```python
from build123d import *

# Parameters (mm, degrees)
SKETCH1_W                = 15.875
SKETCH1_H                = 15.875
BOSS_EXTRUDE1_DEPTH      = 25.4
BOSS_EXTRUDE3_DEPTH      = 3.175
BOSS_EXTRUDE3_DEPTH_BACK = 3.175
SKETCH4_R                = 1.190625
CUT_EXTRUDE1_DEPTH       = 16.875
SKETCH8_R                = 1.5875
CUT_EXTRUDE3_DEPTH       = 7.9375
SKETCH7_R                = 1.5875
CUT_EXTRUDE4_DEPTH       = 7.9375
SKETCH9_W                = 9.525
SKETCH9_H                = 4.7625
CUT_EXTRUDE5_DEPTH       = 26.4
CUT_EXTRUDE6_DEPTH       = 12.1125


with BuildPart() as part:
    # Sketch1 → Boss-Extrude1 (new body)
    with BuildSketch(Plane.XY):
        Rectangle(SKETCH1_W, SKETCH1_H)
    extrude(amount=BOSS_EXTRUDE1_DEPTH)

    # Sketch3 → Boss-Extrude3 (add, two sides)
    with BuildSketch(Plane(origin=(0, 0, 0), x_dir=(1, 0, 0), z_dir=(0, 1, 0))) as boss_extrude3_sk:
        with BuildLine():
            Line((-7.9375, 0), (7.9375, 0))
            ThreePointArc((7.9375, 0), (0, 7.9375), (-7.9375, 0))
        make_face()
    extrude(amount=BOSS_EXTRUDE3_DEPTH)
    extrude(boss_extrude3_sk.sketch, amount=-BOSS_EXTRUDE3_DEPTH_BACK)

    # Sketch4 → Cut-Extrude1 (cut, through all)
    with BuildSketch(Plane(origin=(7.9375, 0, 0), x_dir=(0, 0, -1), z_dir=(1, 0, 0))):
        with Locations((-12.7, 0)):
            Circle(SKETCH4_R)
    extrude(amount=-CUT_EXTRUDE1_DEPTH, mode=Mode.SUBTRACT)

    # Sketch8 → Cut-Extrude3 (cut)
    with BuildSketch(Plane(origin=(6.380613831, 0, -4.72140587), x_dir=(-0.594822787, 0, -0.803856861), z_dir=(0.803856861, 0, -0.594822787))):
        Circle(SKETCH8_R)
    extrude(amount=-CUT_EXTRUDE3_DEPTH, mode=Mode.SUBTRACT)

    # Sketch7 → Cut-Extrude4 (cut)
    with BuildSketch(Plane(origin=(-4.72140587, 0, -6.380613831), x_dir=(0.803856861, 0, -0.594822787), z_dir=(0.594822787, 0, 0.803856861))):
        Circle(SKETCH7_R)
    extrude(amount=CUT_EXTRUDE4_DEPTH, mode=Mode.SUBTRACT)

    # Sketch9 → Cut-Extrude5 (cut, through all)
    with BuildSketch(Plane(origin=(0, 0, 0), x_dir=(-1, 0, 0), z_dir=(0, 0, -1))):
        with Locations((0, 5.55625)):
            Rectangle(SKETCH9_W, SKETCH9_H)
        with Locations((0, -5.55625)):
            Rectangle(SKETCH9_W, SKETCH9_H)
    extrude(amount=-CUT_EXTRUDE5_DEPTH, mode=Mode.SUBTRACT)

    # Sketch10 → Cut-Extrude6 (cut, through all)
    with BuildSketch(Plane(origin=(0, -3.175, 0), x_dir=(-1, 0, 0), z_dir=(0, -1, 0))):
        with BuildLine():
            Line((-3.175, -19.05), (-3.175, -6.35))
            ThreePointArc((-3.175, -6.35), (0, -3.175), (3.175, -6.35))
            Line((3.175, -6.35), (3.175, -19.05))
            ThreePointArc((3.175, -19.05), (0, -22.225), (-3.175, -19.05))
        make_face()
    extrude(amount=-CUT_EXTRUDE6_DEPTH, mode=Mode.SUBTRACT)


solid = part.part
```
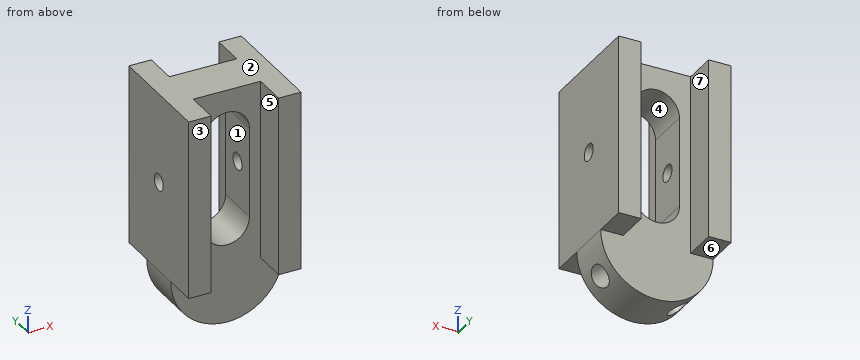
Source: CAD feature listing. Evaluate the final solid. Frame: model axes, mm. Face numbers are marked on the shaded views. A direction names the side the tool comes from. Coordinates: 2 decimals unless noted, no trailing zeros. Loops run counter-clockwise (first coordinate to the right, second up) from the corner with the lowest first, then second, coordinate; pieces in that order, holes last. Notation, with made-up numbers: (78.5, 48.25) -> (108.5, 48.25) arc R20 ccw to (108.5, 66.25) -> close; hole circle Ø11 at (40, 45). An arc over 180 degrees is marked (long way). One line per item, written item: value. Start each with the question number.
Q1. Section query D-D, the plane y = 0. Give the number of separate pieces and of enclosed holes in the cut face, and give its area (3 significant figures).
Q2. Section query C-C, the plane z = 8. Return the cut outline in (x, y) (1 decimal), and give its area (3 significant figures).
Q3. Contact query for flat-ended pins moving along their axis: P1, Ø5, axis at x = -1.5, y = -5.5, coming from the -Z side; P2, Ø5, axis at x = 1, z = 5, coming from the -Y side (3 decimals); P3, Ø1, axis at x = 7, y = 6, coming from the -Z side; P4, Ø2, axis at y = 0, z = 12.7, coming from the +X side. Output: stop coordinate, or through.
Q4. Set-up query: the marked faces 4, 5, 6 and 7. Return all of +Z, -Z, +X, -X, +Y, -Y with unobstructed straight access to the full face (end or side cutting, diameter ignored); none if empty.
Q5. Line query: line 1 along X through (y, z) = (-1.75, 19) (1 decimal); line 2 along X through (y, z) = (-6, 13); line 3 along Z through (x, y) = (1, -0.25). Output: solid intervals per line, ascending.
Q6. Section query B-B, the plane z = 12.7. Return the cut outline in (x, y) (1 decimal).
Q7. Section query A-A, the plane y = -6.25. Return the cut outline in (x, z).
Q8. Mould query, pull axis Z, two halves, no side actions, for the marked faces 1, 2 and 3. Classes: pulls with the +Z half, pulls with the -Z half, needs draft (parallel to the pull), parting line crosses it, or undercut.
Results:
1. separate pieces: 3
1. enclosed holes: 0
1. area: 320 mm^2
2. outline: (-7.9, -7.9) -> (-4.8, -7.9) -> (-4.8, -3.2) -> (-3.2, -3.2) -> (-3.2, 3.2) -> (-4.8, 3.2) -> (-4.8, 7.9) -> (-7.9, 7.9) -> close; (3.2, -3.2) -> (4.8, -3.2) -> (4.8, -7.9) -> (7.9, -7.9) -> (7.9, 7.9) -> (4.8, 7.9) -> (4.8, 3.2) -> (3.2, 3.2) -> close
2. area: 121 mm^2
3. P1: z = -7.92
3. P2: y = -3.175
3. P3: z = 0
3. P4: through
4. face 4: +Y, -Y
4. face 5: +Z, -Z, -Y
4. face 6: -Z, +X, -X, +Y
4. face 7: +Z, -Z, +Y
5. line 1: -7.9 to -3.2, 3.2 to 7.9
5. line 2: -7.94 to -4.76, 4.76 to 7.94
5. line 3: -7.87 to -2.69, 1.21 to 3.34, 22.06 to 25.4
6. outline: (-7.9, -7.9) -> (-4.8, -7.9) -> (-4.8, -3.2) -> (-3.2, -3.2) -> (-3.2, -1.2) -> (-7.9, -1.2) -> close; (-7.9, 1.2) -> (-3.2, 1.2) -> (-3.2, 3.2) -> (-4.8, 3.2) -> (-4.8, 7.9) -> (-7.9, 7.9) -> close; (3.2, -3.2) -> (4.8, -3.2) -> (4.8, -7.9) -> (7.9, -7.9) -> (7.9, -1.2) -> (3.2, -1.2) -> close; (3.2, 1.2) -> (7.9, 1.2) -> (7.9, 7.9) -> (4.8, 7.9) -> (4.8, 3.2) -> (3.2, 3.2) -> close
7. outline: (-7.94, 0) -> (-4.76, 0) -> (-4.76, 25.4) -> (-7.94, 25.4) -> close; (4.76, 0) -> (7.94, 0) -> (7.94, 25.4) -> (4.76, 25.4) -> close
8. face 1: undercut
8. face 2: pulls with the +Z half
8. face 3: needs draft
